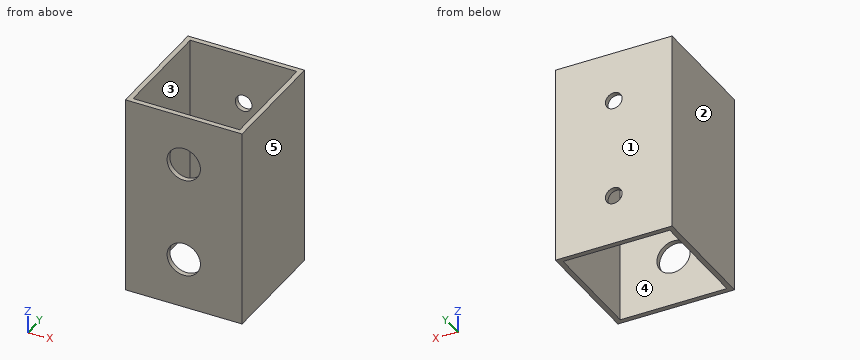
from build123d import *

# Parameters (mm, degrees)
F0_W     = 44.45
F0_H     = 44.45
F0_W_2   = 40.64
F0_H_2   = 40.64
F1_DEPTH = 76.2
F2_R     = 6.35
F3_DEPTH = 25.4
F4_R     = 3.175
F5_DEPTH = 25.4


with BuildPart() as f1:
    # F0 (on Top) → F1 (new body)
    with BuildSketch(Plane.XY):
        Rectangle(F0_W, F0_H)
        Rectangle(F0_W_2, F0_H_2, mode=Mode.SUBTRACT)
    extrude(amount=F1_DEPTH)

    # F2 (on face) → F3 (cut)
    with BuildSketch(Plane.XZ.offset(22.225)):
        with Locations((0, 57.15)):
            Circle(F2_R)
        with Locations((0, 19.05)):
            Circle(F2_R)
    extrude(amount=-F3_DEPTH, mode=Mode.SUBTRACT)

    # F4 (on face) → F5 (cut)
    with BuildSketch(Plane(origin=(0, 22.225, 0), x_dir=(-1, 0, 0), z_dir=(0, 1, 0))):
        with Locations((0, 57.15)):
            Circle(F4_R)
        with Locations((0, 19.05)):
            Circle(F4_R)
    extrude(amount=-F5_DEPTH, mode=Mode.SUBTRACT)


solid = f1.part
Design review of the part built by this model. Coordinates are the model's own, in mm. Face numbers are marked on the shaded views. A direction names the side the tool comes from. Coordinates: 2 decimals unless noted, no trailing zeros. Write each loop counter-clockwise with the first axis right and the second up, starting at its lowest first coordinate (ties: lowest second). Pieces come first, ordered by that corner, then holes. Notation, with made-up numbers: (85.25, -34) - (141.25, -34) arc R18 cw to (141.25, 1) - close; hole circle Ø4 at (-33.75, 87). An arc over 180 degrees is marked (long way). Use one line per item in the form item = value.
Q1. Consider section B-B (y = 0). Write out the cut boundary in (x, z) (3 decimals), plus the area to 3 significant figures.
Taken from the geometry:
outline = (-22.225, 0) - (-20.32, 0) - (-20.32, 76.2) - (-22.225, 76.2) - close; (20.32, 0) - (22.225, 0) - (22.225, 76.2) - (20.32, 76.2) - close
area = 290 mm^2
Q2. Consider section D-D (z = 66.5). Write out the cut boundary in (x, y) (3 decimals), plus the area to 3 significant figures.
Taken from the geometry:
outline = (-22.225, -22.225) - (22.225, -22.225) - (22.225, 22.225) - (-22.225, 22.225) - close; hole (-20.32, -20.32) - (20.32, -20.32) - (20.32, 20.32) - (-20.32, 20.32) - close
area = 324 mm^2
Q3. The part is to be moulded in two halves that separate along X. For the marked faces 1, 2 and 3, say which applies: +X half, -X half, draft (parallel to the pull), parting line (faces both ways), or undercut.
Taken from the geometry:
face_1 = draft
face_2 = -X half
face_3 = undercut
Q4. For probe 1 along Z at (x, y) = (0, 21.5) (3 decimals); probe 2 along Z at (x, y) = (0, -21.5); probe 3 along Y at (x, z) = (14, 20) (3 decimals), list the stretches that pass through material, from the lowest coordinate up.
Taken from the geometry:
probe_1 = 0 to 15.875, 22.225 to 53.975, 60.325 to 76.2
probe_2 = 0 to 12.7, 25.4 to 50.8, 63.5 to 76.2
probe_3 = -22.225 to -20.32, 20.32 to 22.225
Q5. Machinability: for the marked faces 4 and 5, which of the approach directions +Z, -Z, +X, -X, +Y, -Y give a long, thin tool a straight path to every point of the face, cutting with its end or side? Answer none if there is none.
Taken from the geometry:
face_4 = +Z, -Z
face_5 = +Z, -Z, +X, +Y, -Y
Q6. Insertion check: pin 1 Ø3 at (x, z) = (-4, 61.5) entering from -Y (3 decimals); pin 2 Ø10 at (x, z) = (0, 19.05) entering from -Y. Each pin has a flat end and moves straight along its axis. Give the tip position at first contact, or say it passes through.
Taken from the geometry:
pin_1 = -22.225
pin_2 = 20.32
Q7. Consider section A-A (z = 57.15). Write out the cut boundary in (x, y) (3 decimals), plus the area to 3 significant figures.
Taken from the geometry:
outline = (-22.225, -22.225) - (-6.35, -22.225) - (-6.35, -20.32) - (-20.32, -20.32) - (-20.32, 20.32) - (-3.175, 20.32) - (-3.175, 22.225) - (-22.225, 22.225) - close; (3.175, 20.32) - (20.32, 20.32) - (20.32, -20.32) - (6.35, -20.32) - (6.35, -22.225) - (22.225, -22.225) - (22.225, 22.225) - (3.175, 22.225) - close
area = 288 mm^2
